from build123d import *

# Parameters (mm, degrees)
CYLINDER003_R     = 25.4
CYLINDER003_DEPTH = 3.17
CYLINDER001_R     = 12.7
CYLINDER001_DEPTH = 69.85
CYLINDER004_R     = 25.4
CYLINDER004_DEPTH = 3.17


with BuildPart() as cylinder003:
    # Cylinder003 → Cylinder003 (new body)
    with BuildSketch(Plane.XY):
        Circle(CYLINDER003_R)
    extrude(amount=CYLINDER003_DEPTH)


with BuildPart() as cylinder001:
    # Cylinder001 → Cylinder001 (new body)
    with BuildSketch(Plane.XY):
        Circle(CYLINDER001_R)
    extrude(amount=CYLINDER001_DEPTH)


with BuildPart() as fusion:
    # Cylinder004 → Cylinder004 (new body)
    with BuildSketch(Plane.XY.offset(69.85)):
        Circle(CYLINDER004_R)
    extrude(amount=CYLINDER004_DEPTH)

    # Fusion: union Cylinder003, Cylinder001
    add(cylinder003.part)
    add(cylinder001.part)


solid = fusion.part
For this review, take the finished solid that the model builds, in its own axes (mm). A direction names the side the tool comes from. Give positions to 0.01 mm unless a question says otherwise; leave off trailing zeros. Order: outer loops, then holes, each group sorted by start corner. A loop starts at its lowest first (then second) coordinate and runs counter-clockwise, first axis right, second up. Notation, with made-up numbers: M 26.25,30.5 L 71.25,30.5 A15 cw 71.25,53.5 Z; hole C -16.5,13.25 d2. An arc over 180 degrees is marked long. Answer in a Markdown table with one row per item. Add a question column.
(1) Wall thickness on probe 1 along Z at (x, y) = (-4.5, -16); probe 2 along X at (y, z) = (-0.5, 67); probe 3 along Y at (x, z) = (0, 43.5): over which ranges is each line inside the solid? List them lowest first. Write a range as [from, to].
(2) Consider section D-D on z = 15. State the section outline as (x, y) points.
(3) For faces 5 (the face through (-5.506, -24.796, 1.563)), 6 (the face through (5, 12, 3.17)), list the 3-axis set-ups (+Z, -Z, +X, -X, +Y, -Y) from which the entire face can be reached by the end or side of a thin tool; tool diameter is ignored.
(4) Consider section B-B on y = 0. State the section outline as (x, z) points.
(5) Consider section A-A on x = 15.5. State the section outline as (y, z) points.
(6) Mouldability with a two-part tool opening along Z and no side actions: class faces 1 (the face through (0, 0, 73.02)), 2 (the face through (5, 12, 69.85)), 3 (the face through (0, 0, 0)), 4 (the face through (-5.506, -24.796, 71.413)) as +Z half, -Z half, draft (parallel to the pull), parting line (faces both ways), or undercut.
(7) For pin 1 (10 mm diameter, centred on x = -0.5, y = -4, fed in from -Z); pin 2 (12 mm diameter, centred on y = -10, z = 65, fed in from -X); pin 3 (3 mm diameter, centred on y = 1.5, z = 20.5, fed in from -X), all flat-tipped, find the tip position at first contact; note any pin that passes through.
Evaluation:
| question | item | result |
|---|---|---|
| 1 | probe 1 | z = [0, 3.17], [69.85, 73.02] |
| 1 | probe 2 | x = [-12.69, 12.69] |
| 1 | probe 3 | y = [-12.7, 12.7] |
| 2 | outline | C 0,0 d25.4 |
| 3 | face 5 | +Z, -Z |
| 3 | face 6 | none |
| 4 | outline | M -25.4,0 L 25.4,0 L 25.4,3.17 L 12.7,3.17 L 12.7,69.85 L 25.4,69.85 L 25.4,73.02 L -25.4,73.02 L -25.4,69.85 L -12.7,69.85 L -12.7,3.17 L -25.4,3.17 Z |
| 5 | outline | M -20.12,0 L 20.12,0 L 20.12,3.17 L -20.12,3.17 Z; M -20.12,69.85 L 20.12,69.85 L 20.12,73.02 L -20.12,73.02 Z |
| 6 | face 1 | +Z half |
| 6 | face 2 | undercut |
| 6 | face 3 | -Z half |
| 6 | face 4 | draft |
| 7 | pin 1 | stops at z = 0 |
| 7 | pin 2 | stops at x = -24.56 |
| 7 | pin 3 | stops at x = -12.7 |
